The listing builds one solid part. Answer for the finished solid, in the listing's coordinates (mm). Face numbers are marked on the shaded views. A direction names the side the tool comes from. Give positions to 0.01 mm unless a question says otherwise; leave off trailing zeros. Write each loop counter-clockwise with the first axis right and the second up, starting at its lowest first coordinate (ties: lowest second). Pieces come first, ordered by that corner, then holes. Notation, with made-up numbers: (26.25, -17) - (46.25, -17) arc R15 cw to (46.25, -3) - close; hole circle Ø5 at (88.25, -18). An arc over 180 degrees is marked (long way). Answer in a Markdown table with one row per item. Add a question column.
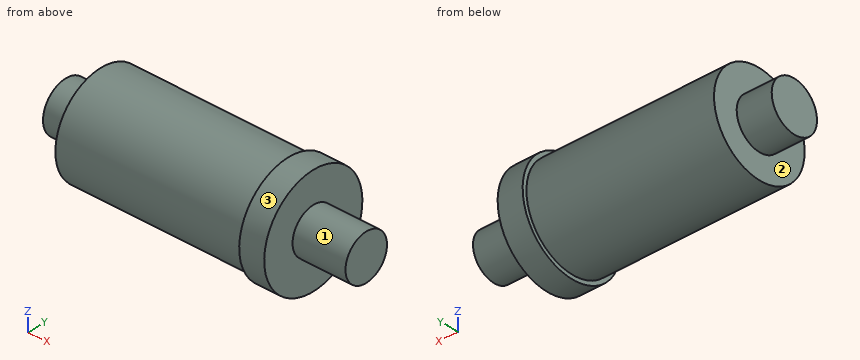
from build123d import *


with BuildPart() as part:
    # Sensor_Turck Sketch → Sensor_Turck (revolve)
    with BuildSketch(Plane.XY, mode=Mode.PRIVATE) as sensor_turck_sk:
        Polygon((12.7, 0), (12.7, 5.5), (0, 5.5), (0, 13), (-6, 13), (-6, 12), (-51, 12), (-51, 6), (-59.4, 6), (-59.4, 0), align=None)
    revolve(sensor_turck_sk.sketch.rotate(Axis((-1000, 0, 0), (1, 0, 0)), 90), axis=Axis((-1000, 0, 0), (1, 0, 0)))


solid = part.part
1. Section C-C (x = -4) is taken. Give the vertices of the cut face in (y, z), and give its area (3 significant figures).
2. Straight lines are drawn through the part: L1, parallel to X at y = -5.5, z = 5.5; L2, parallel to Y at x = -42, z = 0; L3, parallel to Z at x = -46.5, y = -6.25. For each, find the intervals that lie inside material, in ascending order. Write a range as [from, to].
3. Section B-B (y = -7.25) is taken. Give the vertices of the cut face in (x, z), and give its area (3 significant figures).
4. Section A-A (z = 0) is taken. Give the vertices of the cut face in (x, y), and give its area (3 significant figures).
5. A tool of negligible diameter and unlimited length cuts with its end or side. For the marked faces 1, 2 and 3, from which of +Z, -Z, +X, -X, +Y, -Y can it reach the whole face along a straight path? Write none if from no direction.
6. Given pin 1 Ø8 at (x, z) = (-7.5, 8) entering from -Y; pin 2 Ø12 at (x, y) = (-43, 5) entering from -Z; pin 3 Ø4 at (x, z) = (-10.5, 2.5) entering from +Y, each flat-ended and moving along its own axis, determine where each tip first touches the part or whether it passes through.
Geometry check:
| question | item | result |
|---|---|---|
| 1 | outline | circle Ø26 at (0, 0) |
| 1 | area | 531 mm² |
| 2 | L1 | [-51, 0] |
| 2 | L2 | [-12, 12] |
| 2 | L3 | [-10.24, 10.24] |
| 3 | outline | (-51, -9.56) - (-6, -9.56) - (-6, -10.79) - (0, -10.79) - (0, 10.79) - (-6, 10.79) - (-6, 9.56) - (-51, 9.56) - close |
| 3 | area | 990 mm² |
| 4 | outline | (-59.4, -6) - (-51, -6) - (-51, -12) - (-6, -12) - (-6, -13) - (0, -13) - (0, -5.5) - (12.7, -5.5) - (12.7, 5.5) - (0, 5.5) - (0, 13) - (-6, 13) - (-6, 12) - (-51, 12) - (-51, 6) - (-59.4, 6) - close |
| 4 | area | 1,480 mm² |
| 5 | face 1 | +X |
| 5 | face 2 | -X |
| 5 | face 3 | +X, -X |
| 6 | pin 1 | y = -12.27 |
| 6 | pin 2 | z = -12 |
| 6 | pin 3 | y = 11.99 |
